Geometry: final body of the model. Coordinates: model frame, mm. A direction names the side the tool comes from. Give positions to 0.01 mm unless a question says otherwise; leave off trailing zeros. Write each loop counter-clockwise with the first axis right and the second up, starting at its lowest first coordinate (ties: lowest second). Pieces come first, ordered by that corner, then holes. Notation, with made-up numbers: M 15.5,75.25 L 24.5,75.25 A23 cw 24.5,85.25 Z; hole C -12,31 d11. An arc over 180 degrees is marked long. Answer as a JSON object with one key per item and string values.
from build123d import *

# Parameters (mm, degrees)
F1_DEPTH = 7.5
F3_DEPTH = 25
F5_DEPTH = 6
F7_DEPTH = 6
F9_DEPTH = 6


with BuildPart() as f1:
    # F0 (on Top) → F1 (new body)
    with BuildSketch(Plane.XY):
        with BuildLine():
            ThreePointArc((-9.5912313469, -5.5375), (-9.5912313469, 5.5375), (0, 11.075))
            Line((0, 11.075), (0, 16))
            ThreePointArc((0, 16), (-3.3224189775, 15.6512469835), (-6.5, 14.6201915172))
            ThreePointArc((-6.5, 14.6201915172), (-13.8564064606, 8), (-15.9114572621, -1.680930634))
            ThreePointArc((-15.9114572621, -1.680930634), (-15.2155869774, -4.9483242552), (-13.8564064606, -8))
            Line((-13.8564064606, -8), (-9.5912313469, -5.5375))
        make_face()
        with BuildLine():
            ThreePointArc((0, 11.075), (7.8312076016, 7.8312076016), (11.075, 0))
            ThreePointArc((11.075, 0), (10.6976285262, -2.8664209245), (9.5912313469, -5.5375))
            Line((9.5912313469, -5.5375), (13.8564064606, -8))
            ThreePointArc((13.8564064606, -8), (15.2155869774, -4.9483242552), (15.9114572621, -1.680930634))
            ThreePointArc((15.9114572621, -1.680930634), (15.9778489822, -0.8416305028), (16, 0))
            ThreePointArc((16, 0), (13.416407865, 8.7177978871), (6.5, 14.6201915172))
            ThreePointArc((6.5, 14.6201915172), (3.3224189775, 15.6512469835), (0, 16))
            Line((0, 16), (0, 11.075))
        make_face()
        with BuildLine():
            Line((13.8564064606, -8), (9.5912313469, -5.5375))
            ThreePointArc((9.5912313469, -5.5375), (0, -11.075), (-9.5912313469, -5.5375))
            Line((-9.5912313469, -5.5375), (-13.8564064606, -8))
            ThreePointArc((-13.8564064606, -8), (-11.8931679998, -10.7029227283), (-9.4114572621, -12.9392608832))
            ThreePointArc((-9.4114572621, -12.9392608832), (0, -16), (9.4114572621, -12.9392608832))
            ThreePointArc((9.4114572621, -12.9392608832), (11.8931679998, -10.7029227283), (13.8564064606, -8))
        make_face()
        with BuildLine():
            Line((0, 25), (0, 16))
            ThreePointArc((0, 16), (3.3224189775, 15.6512469835), (6.5, 14.6201915172))
            Line((6.5, 14.6201915172), (6.5, 25))
            Line((6.5, 25), (0, 25))
        make_face()
        with BuildLine():
            ThreePointArc((-6.5, 14.6201915172), (-3.3224189775, 15.6512469835), (0, 16))
            Line((0, 16), (0, 25))
            Line((0, 25), (-6.5, 25))
            Line((-6.5, 25), (-6.5, 14.6201915172))
        make_face()
        with BuildLine():
            Line((-21.6506350946, -12.5), (-13.8564064606, -8))
            ThreePointArc((-13.8564064606, -8), (-15.2155869774, -4.9483242552), (-15.9114572621, -1.680930634))
            Line((-15.9114572621, -1.680930634), (-24.9006350946, -6.8708348754))
            Line((-24.9006350946, -6.8708348754), (-21.6506350946, -12.5))
        make_face()
        with BuildLine():
            ThreePointArc((-9.4114572621, -12.9392608832), (-11.8931679998, -10.7029227283), (-13.8564064606, -8))
            Line((-13.8564064606, -8), (-21.6506350946, -12.5))
            Line((-21.6506350946, -12.5), (-18.4006350946, -18.1291651246))
            Line((-18.4006350946, -18.1291651246), (-9.4114572621, -12.9392608832))
        make_face()
        with BuildLine():
            Line((21.6506350946, -12.5), (13.8564064606, -8))
            ThreePointArc((13.8564064606, -8), (11.8931679998, -10.7029227283), (9.4114572621, -12.9392608832))
            Line((9.4114572621, -12.9392608832), (18.4006350946, -18.1291651246))
            Line((18.4006350946, -18.1291651246), (21.6506350946, -12.5))
        make_face()
        with BuildLine():
            ThreePointArc((15.9114572621, -1.680930634), (15.2155869774, -4.9483242552), (13.8564064606, -8))
            Line((13.8564064606, -8), (21.6506350946, -12.5))
            Line((21.6506350946, -12.5), (24.9006350946, -6.8708348754))
            Line((24.9006350946, -6.8708348754), (15.9114572621, -1.680930634))
        make_face()
    extrude(amount=F1_DEPTH)

    # F2 (on face) → F3 (cut)
    with BuildSketch(Plane.XY.offset(7.5)):
        Polygon((5, 22.5), (0, 22.5), (-5, 22.5), (-5, 18.5), (5, 18.5), align=None)
        Polygon((-21.9855715851, -6.9198729811), (-19.4855715851, -11.25), (-16.02146997, -9.25), (-18.52146997, -4.9198729811), align=None)
        Polygon((-16.02146997, -9.25), (-19.4855715851, -11.25), (-16.9855715851, -15.5801270189), (-13.52146997, -13.5801270189), align=None)
        Polygon((16.9855715851, -15.5801270189), (19.4855715851, -11.25), (16.02146997, -9.25), (13.52146997, -13.5801270189), align=None)
        Polygon((16.02146997, -9.25), (19.4855715851, -11.25), (21.9855715851, -6.9198729811), (18.52146997, -4.9198729811), align=None)
    extrude(amount=-F3_DEPTH, mode=Mode.SUBTRACT)

    # F4 (on face) → F5 (cut)
    with BuildSketch(Plane(origin=(21.6506350946, -12.5, 0), x_dir=(0.5, 0.8660254038, 0), z_dir=(0.8660254038, -0.5, 0))):
        with BuildLine():
            ThreePointArc((0, 6.875), (-3.125, 3.75), (0, 0.625))
            Line((0, 0.625), (0, 6.875))
        make_face()
        with BuildLine():
            Line((0, 6.875), (0, 0.625))
            ThreePointArc((0, 0.625), (2.2097086912, 1.5402913088), (3.125, 3.75))
            ThreePointArc((3.125, 3.75), (2.2097086912, 5.9597086912), (0, 6.875))
        make_face()
    extrude(amount=-F5_DEPTH, mode=Mode.SUBTRACT)

    # F6 (on face) → F7 (cut)
    with BuildSketch(Plane(origin=(0, 25, 0), x_dir=(-1, 0, 0), z_dir=(0, 1, 0))):
        with BuildLine():
            Line((0, 6.875), (0, 0.625))
            ThreePointArc((0, 0.625), (2.2097086912, 1.5402913088), (3.125, 3.75))
            ThreePointArc((3.125, 3.75), (2.2097086912, 5.9597086912), (0, 6.875))
        make_face()
        with BuildLine():
            ThreePointArc((0, 6.875), (-3.125, 3.75), (0, 0.625))
            Line((0, 0.625), (0, 6.875))
        make_face()
    extrude(amount=-F7_DEPTH, mode=Mode.SUBTRACT)

    # F8 (on face) → F9 (cut)
    with BuildSketch(Plane(origin=(-21.6506350946, -12.5, 0), x_dir=(0.5, -0.8660254038, 0), z_dir=(-0.8660254038, -0.5, 0))):
        with BuildLine():
            ThreePointArc((3.125, 3.75), (2.2097086912, 5.9597086912), (0, 6.875))
            Line((0, 6.875), (0, 0.625))
            ThreePointArc((0, 0.625), (2.2097086912, 1.5402913088), (3.125, 3.75))
        make_face()
        with BuildLine():
            Line((0, 0.625), (0, 6.875))
            ThreePointArc((0, 6.875), (-3.125, 3.75), (0, 0.625))
        make_face()
    extrude(amount=-F9_DEPTH, mode=Mode.SUBTRACT)


solid = f1.part
1) Cut plane A-A on y = 21.5. Return loops of the section in (x, z), and give its area (3 significant figures).
Geometry check:
{"outline": "M -6.5,0 L -5,0 L -5,7.5 L -6.5,7.5 Z; M 5,0 L 6.5,0 L 6.5,7.5 L 5,7.5 Z", "area": "22.5 mm2"}
2) Contact query for flat-ended pins moving along their axis: P1, Ø2, axis at y = 19.5, z = 4.5, coming from the -X side; P2, Ø2, axis at y = 11, z = 3.5, coming from the +X side; P3, Ø1.2, axis at y = 20, z = 3.5, coming from the +X side. Output: stop coordinate, or through.
Geometry check:
{"P1": "stops at x = -6.5", "P2": "stops at x = 12.49", "P3": "stops at x = 6.5"}
3) Line query: line 1 (Y direction, x = -4, z = 4); line 2 (X direction, y = 20, z = 3.5); line 3 (Y direction, x = 2.5, z = 5.75). Output: solid intervals per line, ascending. Write a range as from..to.
Geometry check:
{"line 1": "y = -15.49..-10.33, 10.33..18.5, 22.5..25", "line 2": "x = -6.5..-5, 5..6.5", "line 3": "y = -15.8..-10.79, 10.79..18.5, 22.5..25"}
4) Pull-direction query (X, two-part tool) for faces 4 (the flat face through (20.469, -4.312, 3.698)), 5 (the flat face through (-6.5, 20, 4)), 6 (the flat face through (17.784, -14.197, 3.802)); classes: pulls with the +X half, pulls with the -X half, needs draft (parallel to the pull), parting line crosses it, or undercut.
Geometry check:
{"face 4": "pulls with the +X half", "face 5": "pulls with the -X half", "face 6": "undercut"}
5) Cut plane B-B on y = 9. Return loops of the section in (x, z), and give its area (3 significant figures).
Geometry check:
{"outline": "M -13.23,0 L -6.45,0 L -6.45,7.5 L -13.23,7.5 Z; M 6.45,0 L 13.23,0 L 13.23,7.5 L 6.45,7.5 Z", "area": "102 mm2"}
6) Set-up query: faces 1 (the flat face through (-13.97, -15.57, 3.7)), 2 (the flat face through (-11, -3, 0)), 3 (the flat face through (16.056, -9.189, 3.802)). Return all of +Z, -Z, +X, -X, +Y, -Y with unobstructed straight access to the full face (end or side cutting, diameter ignored); none if empty.
Geometry check:
{"face 1": "+Z, -Z, -Y", "face 2": "-Z, +X, -X, +Y, -Y", "face 3": "+Z, -Z"}
